Build history of the part. All positions in model axes, mm. A direction names the side the tool comes from. Give positions to 0.01 mm unless a question says otherwise; leave off trailing zeros. Order: outer loops, then holes, each group sorted by start corner. A loop starts at its lowest first (then second) coordinate and runs counter-clockwise, first axis right, second up. Notation, with made-up numbers: M -37.75,27 L 0.25,27 A15 ccw 0.25,33 Z; hole C 28.25,61.5 d9. An arc over 180 degrees is marked long. Answer as CSV lines item,"result".
from build123d import *

# Parameters (mm, degrees)
SKETCH1_W           = 6
SKETCH1_H           = 6
BOSS_EXTRUDE1_DEPTH = 3
SKETCH2_R           = 1.75
BOSS_EXTRUDE2_DEPTH = 1.5
SKETCH3_R           = 0.65
BOSS_EXTRUDE3_DEPTH = 0.5
SKETCH4_W           = 0.64
SKETCH4_H           = 0.64
BOSS_EXTRUDE4_DEPTH = 3.2
FILLET1_R           = 0.4
SKETCH6_W           = 0.64
SKETCH6_H           = 0.64
BOSS_EXTRUDE6_DEPTH = 7.14


with BuildPart() as part:
    # Sketch1 → Boss-Extrude1 (new body)
    with BuildSketch(Plane(origin=(0, 0, 0), x_dir=(1, 0, 0), z_dir=(0, 1, 0))):
        Rectangle(SKETCH1_W, SKETCH1_H)
    extrude(amount=BOSS_EXTRUDE1_DEPTH)

    # Sketch2 → Boss-Extrude2 (add)
    with BuildSketch(Plane(origin=(0, 3, 0), x_dir=(1, 0, 0), z_dir=(0, 1, 0))):
        Circle(SKETCH2_R)
    extrude(amount=BOSS_EXTRUDE2_DEPTH)

    # Sketch3 → Boss-Extrude3 (add)
    with BuildSketch(Plane(origin=(0, 3, 0), x_dir=(1, 0, 0), z_dir=(0, 1, 0))):
        with Locations((-2, 2)):
            Circle(SKETCH3_R)
        with Locations((-2, -2)):
            Circle(SKETCH3_R)
        with Locations((2, -2)):
            Circle(SKETCH3_R)
        with Locations((2, 2)):
            Circle(SKETCH3_R)
    extrude(amount=BOSS_EXTRUDE3_DEPTH)

    # Sketch4 → Boss-Extrude4 (add)
    with BuildSketch(Plane.XZ):
        with Locations((-3.25, 2.25)):
            Rectangle(SKETCH4_W, SKETCH4_H)
        with Locations((3.25, 2.25)):
            Rectangle(SKETCH4_W, SKETCH4_H)
        with Locations((3.25, -2.25)):
            Rectangle(SKETCH4_W, SKETCH4_H)
        with Locations((-3.25, -2.25)):
            Rectangle(SKETCH4_W, SKETCH4_H)
    extrude(amount=BOSS_EXTRUDE4_DEPTH)

    # Fillet1
    fillet1_edges = [part.edges().sort_by_distance(p)[0] for p in [
        (3, 1.5, 3),
        (-3, 1.5, 3),
        (-3, 1.5, -3),
        (3, 1.5, -3),
    ]]
    fillet(fillet1_edges, radius=FILLET1_R)

    # Sketch6 → Boss-Extrude6 (add)
    with BuildSketch(Plane.ZY.offset(3.57)):
        with Locations((-2.25, 0.32)):
            Rectangle(SKETCH6_W, SKETCH6_H)
        with Locations((2.25, 0.32)):
            Rectangle(SKETCH6_W, SKETCH6_H)
    extrude(amount=-BOSS_EXTRUDE6_DEPTH)


solid = part.part
Item 1: 3-axis set-ups, long thin cutter, end or side, ignore diameter. For faces 1 (the flat face through (2, 3.5, 2)), 2 (the cylindrical face through (2.6, 3.25, 2.25)), 3 (the flat face through (-2, 3.5, -2)): which of +Z, -Z, +X, -X, +Y, -Y reach the whole face in a straight line?
Geometry says:
face 1,"+Z, +X, +Y"
face 2,"+Y"
face 3,"-Z, -X, +Y"
Item 2: Band-saw the part on D-D (x = 0). Give the cut face in (y, z), and give its area (4 significant figures).
Geometry says:
outline,"M 0,-3 L 3,-3 L 3,-1.75 L 4.5,-1.75 L 4.5,1.75 L 3,1.75 L 3,3 L 0,3 Z"
area,"23.25 mm2"
Item 3: Pull direction X, two halves, no side cores. Call faces 4 (the flat face through (0, 0, 0)), 5 (the flat face through (0, 4.5, 0)): released by +X, released by -X, zero draft, split by the parting line, or undercut.
Geometry says:
face 4,"undercut"
face 5,"zero draft"
Item 4: Band-saw the part on B-B (x = 2.25). Give the cut face in (y, z), and give its area (3 significant figures).
Geometry says:
outline,"M 0,-3 L 3,-3 L 3,-2.6 L 3.5,-2.6 L 3.5,-1.4 L 3,-1.4 L 3,1.4 L 3.5,1.4 L 3.5,2.6 L 3,2.6 L 3,3 L 0,3 Z"
area,"19.2 mm2"
Item 5: Drop flat-ended pins along their axis: pin 1 (1.4 mm diameter, centred on x = -2, z = 2, fed in from +Y); pin 2 (2.5 mm diameter, centred on y = 1, z = 0, fed in from -X); pin 3 (0.7 mm diameter, centred on x = -3, y = -1.5, fed in from +Z). Give the stop position or say it passes through.
Geometry says:
pin 1,"stops at y = 3.5"
pin 2,"stops at x = -3"
pin 3,"stops at z = 2.57"
Item 6: Band-saw the part on C-C (z = 0.7). Give the cut face in (x, y), and give its area (3 significant figures).
Geometry says:
outline,"M -3,0 L 3,0 L 3,3 L 1.6,3 L 1.6,4.5 L -1.6,4.5 L -1.6,3 L -3,3 Z"
area,"22.8 mm2"
Item 7: Band-saw the part on A-A (y = -0.5). Give the cut face in (x, z).
Geometry says:
outline,"M -3.57,-2.57 L -2.93,-2.57 L -2.93,-1.93 L -3.57,-1.93 Z; M -3.57,1.93 L -2.93,1.93 L -2.93,2.57 L -3.57,2.57 Z; M 2.93,-2.57 L 3.57,-2.57 L 3.57,-1.93 L 2.93,-1.93 Z; M 2.93,1.93 L 3.57,1.93 L 3.57,2.57 L 2.93,2.57 Z"
Item 8: Probe line 1 along X through (y, z) = (-1.5, 2.1); line 2 along Y through (x, z) = (-1.25, 0.7); line 3 along X through (y, z) = (1.75, -0.25). List the from-to ranges inside material, lowest first. Write a range as from..to.
Geometry says:
line 1,"x = -3.57..-2.93, 2.93..3.57"
line 2,"y = 0..4.5"
line 3,"x = -3..3"
